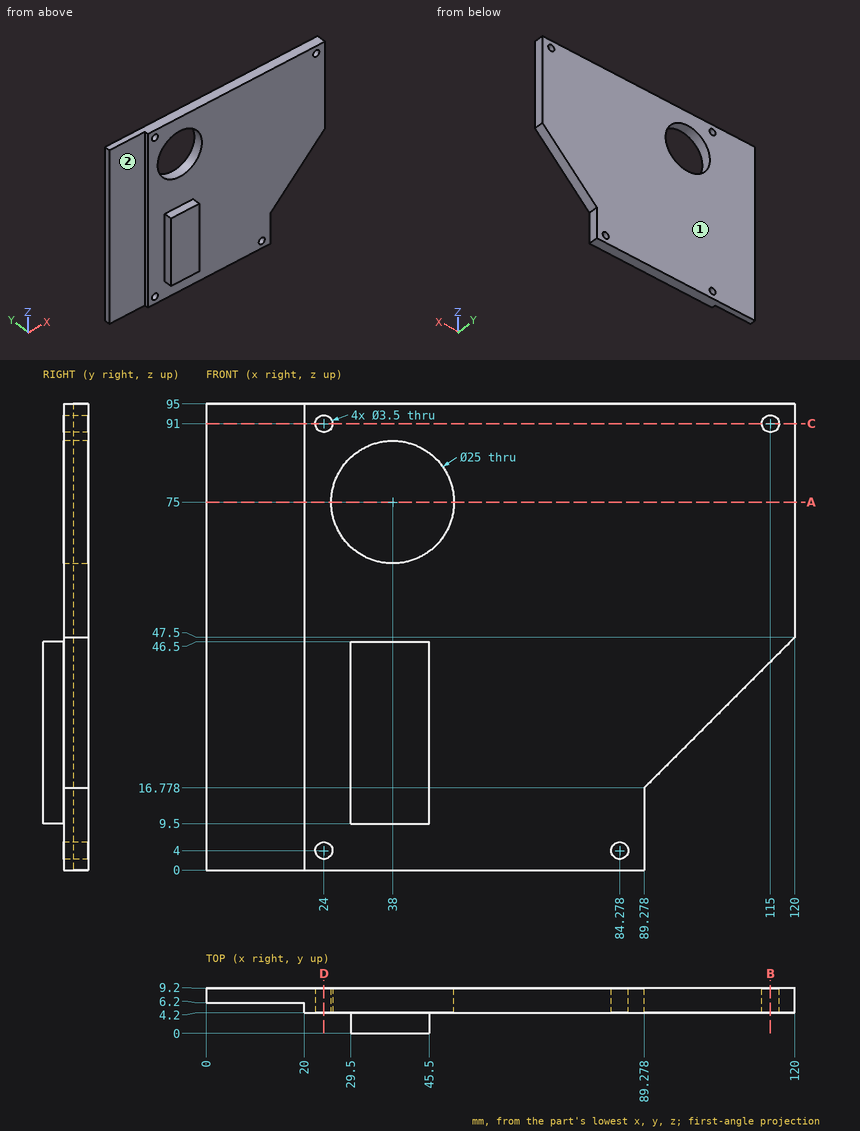
Geometry check sheet. Reference: drawing and pictorial views, mm from the part's lowest x, y, z. A direction names the side the tool comes from. Coordinates: 2 decimals unless noted, no trailing zeros. Order: outer loops, then holes, each group sorted by start corner. A loop starts at its lowest first (then second) coordinate and runs counter-clockwise, first axis right, second up.
1. Go/stop test with flat-tipped pins: pin 1 Ø2 at (y, z) = (1.5, 19.5) entering from -X; pin 2 Ø2 at (y, z) = (2.5, 25) entering from +X; pin 3 Ø4.5 at (x, z) = (24, 91) entering from -Y. Record where each tip stops, or that it passes through.
Results found:
pin 1: stops at x = 29.5
pin 2: stops at x = 45.5
pin 3: stops at y = 4.2
2. Sectioned sample at A-A, the plane z = 75. Record the cut outline in (x, y), and give its area (3 significant figures).
Results found:
outline: (0, 6.2) - (20, 6.2) - (20, 4.2) - (25.5, 4.2) - (25.5, 9.2) - (0, 9.2) - close; (50.5, 4.2) - (120, 4.2) - (120, 9.2) - (50.5, 9.2) - close
area: 435 mm2
3. Set-up check for the marked faces 1 and 2: record each of +Z, -Z, +X, -X, +Y, -Y from which the full face is reachable in a straight line by a thin tool's end or side.
Results found:
face 1: +Z, -Z, +X, -X, +Y
face 2: +Z, -Z, -X, -Y
4. Scan lines: line 1 (X direction, y = 7.75, z = 91); line 2 (Z direction, x = 24, y = 7.8); line 3 (X direction, y = 6.55, z = 4). Record each from-to range of solid material in increasing order.
Results found:
line 1: x = 0 to 22.25, 25.75 to 113.25, 116.75 to 120
line 2: z = 0 to 2.25, 5.75 to 89.25, 92.75 to 95
line 3: x = 0 to 22.25, 25.75 to 82.53, 86.03 to 89.28
5. Sectioned sample at D-D, the plane x = 24. Record the cut outline in (y, z), and give its area (3 significant figures).
Results found:
outline: (4.2, 0) - (9.2, 0) - (9.2, 2.25) - (4.2, 2.25) - close; (4.2, 5.75) - (9.2, 5.75) - (9.2, 89.25) - (4.2, 89.25) - close; (4.2, 92.75) - (9.2, 92.75) - (9.2, 95) - (4.2, 95) - close
area: 440 mm2
6. Sectioned sample at C-C, the plane z = 91. Record the cut outline in (x, y).
Results found:
outline: (0, 6.2) - (20, 6.2) - (20, 4.2) - (22.25, 4.2) - (22.25, 9.2) - (0, 9.2) - close; (25.75, 4.2) - (113.25, 4.2) - (113.25, 9.2) - (25.75, 9.2) - close; (116.75, 4.2) - (120, 4.2) - (120, 9.2) - (116.75, 9.2) - close
7. Sectioned sample at B-B, the plane x = 115. Record the cut outline in (y, z), and give its area (3 significant figures).
Results found:
outline: (4.2, 42.5) - (9.2, 42.5) - (9.2, 89.25) - (4.2, 89.25) - close; (4.2, 92.75) - (9.2, 92.75) - (9.2, 95) - (4.2, 95) - close
area: 245 mm2
